Autodesk Inventor part; units mm, degrees
ref_plane "YZ Plane" through (0, 0, 0) normal (1, 0, 0) x (0, 1, 0)
ref_plane "XZ Plane" through (0, 0, 0) normal (0, 1, 0) x (-1, 0, 0)
ref_plane "XY Plane" through (0, 0, 0) normal (0, 0, 1) x (1, 0, 0)
sketch "Sketch1" plane through (0, 0, 0) normal (0, 0, 1) x (1, 0, 0)
  line L0 (-30, 44) -> (-30, 64)
  line L1 (-30, 64) -> (-2, 64)
  line L2 (-2, 64) -> (-2, 44)
  line L3 (-2, 44) -> (-30, 44)
  line L4 (-61.5, 40) -> (-61.5, 60)
  line L5 (-61.5, 60) -> (-46.5, 60)
  line L6 (-46.5, 60) -> (-46.5, 40)
  line L7 (-46.5, 40) -> (-61.5, 40)
  line L8 (-53, 6.2) -> (-53, 16.8)
  line L9 (-53, 16.8) -> (-29, 16.8)
  line L10 (-29, 16.8) -> (-29, 6.2)
  line L11 (-29, 6.2) -> (-53, 6.2)
  line L12 (-29, 70.2) -> (-29, 80.8)
  line L13 (-29, 80.8) -> (-5, 80.8)
  line L14 (-5, 80.8) -> (-5, 70.2)
  line L15 (-5, 70.2) -> (-29, 70.2)
  line L16 (-58, 70.2) -> (-58, 80.8)
  line L17 (-58, 80.8) -> (-34, 80.8)
  line L18 (-34, 80.8) -> (-34, 70.2)
  line L19 (-34, 70.2) -> (-58, 70.2)
  circle A0 centre (-3, 19.5) radius 1.5
  circle A1 centre (-9.5, 19.5) radius 1.5
  circle A2 centre (-26.5, 18.5) radius 1.5
  circle A3 centre (-26.5, 4.5) radius 1.5
  circle A4 centre (-55.5, 4.5) radius 1.5
  circle A5 centre (-55.5, 18.5) radius 1.5
  circle A6 centre (-2.5, 68.5) radius 1.5
  circle A7 centre (-60.5, 68.5) radius 1.5
  circle A8 centre (-60.5, 82.5) radius 1.5
  circle A9 centre (-2.5, 82.5) radius 1.5
  circle A10 centre (-54, 37) radius 0.75
  circle A11 centre (-54, 63) radius 0.75
  arc A12 (-63, 26.3448) -> (-60.5004, 22.6368) centre (-59, 26.3448) ccw
  arc A13 (-58.0008, 18.9289) -> (-60.5004, 22.6368) centre (-62.0008, 18.9289) ccw
  line L20 (-58.0008, 18.9289) -> (-58.0008, 4)
  arc A14 (-58.0008, 4) -> (-54.0008, 0) centre (-54.0008, 4) ccw
  line L21 (-54.0008, 0) -> (-24, 0)
  line L22 (-24, 0) -> (-24, 6.4)
  line L23 (-24, 6.4) -> (-21, 6.4)
  line L24 (-21, 6.4) -> (-21, 33.4)
  line L25 (-21, 33.4) -> (-15, 33.4)
  line L26 (-15, 33.4) -> (-15, 6.4)
  line L27 (-15, 6.4) -> (-9, 6.4)
  line L28 (-9, 6.4) -> (-9, 13.4)
  line L29 (-9, 13.4) -> (-10.25, 13.4)
  line L30 (-10.25, 13.4) -> (-10.25, 15.2)
  line L31 (-10.25, 15.2) -> (-9, 15.2)
  line L32 (-9, 15.2) -> (-9, 17)
  line L33 (-9, 17) -> (-6, 17)
  line L34 (-6, 17) -> (-6, 15.2)
  line L35 (-6, 15.2) -> (-4.75, 15.2)
  line L36 (-4.75, 15.2) -> (-4.75, 13.4)
  line L37 (-4.75, 13.4) -> (-6, 13.4)
  line L38 (-6, 13.4) -> (-6, 6.4)
  line L39 (-6, 6.4) -> (0, 6.4)
  line L40 (0, 6.4) -> (0, 47)
  arc A15 (4, 51) -> (0, 47) centre (4, 47) ccw
  line L41 (7, 51) -> (4, 51)
  line L42 (7, 73) -> (7, 51)
  line L43 (4, 73) -> (7, 73)
  arc A16 (0, 77) -> (4, 73) centre (4, 77) ccw
  line L44 (0, 77) -> (0, 83)
  arc A17 (0, 83) -> (-4, 87) centre (-4, 83) ccw
  line L45 (-4, 87) -> (-59, 87)
  arc A18 (-59, 87) -> (-63, 83) centre (-59, 83) ccw
  line L46 (-63, 83) -> (-63, 26.3448)
  point P0 (0, 0)
  point P1 (0, 0)
extrude "Extrusion1" add sketch "Sketch1" along normal blind 6
properties part number "yCarBottom"
Can you work these out from the model? Positions are in its coordinate system, mm. A direction names the side the tool comes from. Coordinates: 2 decimals unless noted, no trailing zeros. Order: outer loops, then holes, each group sorted by start corner. A loop starts at its lowest first (then second) coordinate and runs counter-clockwise, first axis right, second up. Notation, with made-up numbers: (37.5, -21.5) - (44.5, -21.5) arc R20 cw to (44.5, -16.5) - close; hole circle Ø9 at (3.25, 64). An arc over 180 degrees is marked (long way). Answer in a Markdown table with one row per item.
1. For pin 1 (3 mm diameter, centred on y = 3, z = 3, fed in from +X); pin 2 (3 mm diameter, centred on y = 11, z = 1.5, fed in from -X), each with a flat end and sliding along its axis, tell me the tip position at first contact or that it passes through.
Reply:
| item | result |
|---|---|
| pin 1 | stops at x = -24 |
| pin 2 | stops at x = -58 |
2. Suppose I cut it at A-A (x = -42). Please give me the cut outline in (y, z), and give its area (3 significant figures).
Reply:
| item | result |
|---|---|
| outline | (0, 0) - (6.2, 0) - (6.2, 6) - (0, 6) - close; (16.8, 0) - (70.2, 0) - (70.2, 6) - (16.8, 6) - close; (80.8, 0) - (87, 0) - (87, 6) - (80.8, 6) - close |
| area | 395 mm^2 |
3. For faces 1 (the flat face through (7, 62, 3)), 2 (the flat face through (0, 26, 3)), 3 (the flat face through (-9, 16, 3)), 4 (the flat face through (-46, 70.2, 3)), 5 (the cylindrical face through (-61.859, 85.797, 2.958)), which set-ups out of +Z, -Z, +X, -X, +Y, -Y let a thin tool reach every point of the face, with its end or its side?
Reply:
| item | result |
|---|---|
| face 1 | +Z, -Z, +X, +Y, -Y |
| face 2 | +Z, -Z, +X, -Y |
| face 3 | +Z, -Z, -Y |
| face 4 | +Z, -Z |
| face 5 | +Z, -Z, -X, +Y |
4. If we mould it in two halves opening along X, with no side actions, what happens to faces 6 (the cylindrical face through (-1.203, 85.859, 2.958)), 7 (the flat face through (-36, 44, 0)), 8 (the flat face through (-29, 75, 3))? For each: pulls with the +X half, pulls with the -X half, needs draft (parallel to the pull), parting line crosses it, or undercut.
Reply:
| item | result |
|---|---|
| face 6 | pulls with the +X half |
| face 7 | needs draft |
| face 8 | undercut |
5. If I drill on line 1 along X through (y, z) = (57, 5.7); line 2 along Y through (x, z) = (-26.5, 3.5); line 3 along Y through (x, z) = (-43, 4.9), over which ranges is the centre line in solid material (lowest first)?
Reply:
| item | result |
|---|---|
| line 1 | x = -63 to -61.5, -46.5 to -30, -2 to 7 |
| line 2 | y = 0 to 3, 6 to 17, 20 to 44, 64 to 70.2, 80.8 to 87 |
| line 3 | y = 0 to 6.2, 16.8 to 70.2, 80.8 to 87 |
6. Suppose I cut it at C-C (y = 54). Please give me the cut outline in (x, z), and give its area (3 significant figures).
Reply:
| item | result |
|---|---|
| outline | (-63, 0) - (-61.5, 0) - (-61.5, 6) - (-63, 6) - close; (-46.5, 0) - (-30, 0) - (-30, 6) - (-46.5, 6) - close; (-2, 0) - (7, 0) - (7, 6) - (-2, 6) - close |
| area | 162 mm^2 |
7. Suppose I cut it at B-B (y = 11.5). Please give me the cut outline in (x, z).
Reply:
| item | result |
|---|---|
| outline | (-58, 0) - (-53, 0) - (-53, 6) - (-58, 6) - close; (-29, 0) - (-21, 0) - (-21, 6) - (-29, 6) - close; (-15, 0) - (-9, 0) - (-9, 6) - (-15, 6) - close; (-6, 0) - (0, 0) - (0, 6) - (-6, 6) - close |
8. Suppose I cut it at D-D (x = -26.5). Please give me the cut outline in (y, z), and give its area (3 significant figures).
Reply:
| item | result |
|---|---|
| outline | (0, 0) - (3, 0) - (3, 6) - (0, 6) - close; (6, 0) - (17, 0) - (17, 6) - (6, 6) - close; (20, 0) - (44, 0) - (44, 6) - (20, 6) - close; (64, 0) - (70.2, 0) - (70.2, 6) - (64, 6) - close; (80.8, 0) - (87, 0) - (87, 6) - (80.8, 6) - close |
| area | 302 mm^2 |
